Check sheet for the modelled part. Datum: model origin and axes. Units: mm. A direction names the side the tool comes from. Round coordinates to 2 decimals unless told otherwise and drop trailing zeros. Loops run counter-clockwise (first coordinate to the right, second up) from the corner with the lowest first, then second, coordinate; pieces in that order, holes last. Notation, with made-up numbers: (80, 67) - (111, 67) arc R14 ccw to (111, 90) - close; hole circle Ø3 at (61.5, 43). An arc over 180 degrees is marked (long way). Answer in a Markdown table with one row per item. Add a question column.
(1) Access from +Z, -Z, +X, -X, +Y, -Y to the whole of each face (thin tool, end or side, straight path). Record for faces 1 (the cylindrical face through (1, 1.05, 4.03)), 2 (the flat face through (19.8, 35, 3.5)).
(2) Thickness scan on line 1 along Y through (x, z) = (36.5, 3.65); line 2 along Y through (x, z) = (18, 5.55); line 3 along X through (y, z) = (32, 3.55). Record the ranges inside material, lowest first.
(3) Gauge pin test, flat end, axial feed: pin 1 (0.9 mm diameter, centred on x = 37, y = 36, fed in from +Z). Record the tip position at first contact, or that the pin passes through.
(4) Cross-section at B-B on x = 21.5. Enter the section's corners in (y, z).
(5) Cross-section at A-A on z = 4.5. Count the separate pieces of the cut face and the enclosed holes in it, then the cut area to 3 significant figures.
(6) Mould release check, pull along X, two halves, no side actions. Record for faces 3 (the flat face through (36, 37, 2)), 4 (the flat face through (20, 0, 4)), 5 (the cylindrical face through (1, 38.95, 3.97)): +X half, -X half, draft (parallel to the pull), parting line (faces both ways), or undercut.
(7) Cross-section at C-C on y = 6. Enter the section's corners in (x, z).
from build123d import *

# Parameters (mm, degrees)
SKETCH1_W           = 40
SKETCH1_H           = 40
BOSS_EXTRUDE1_DEPTH = 2
SKETCH2_W           = 40
SKETCH2_H           = 40
SKETCH2_W_2         = 30
SKETCH2_H_2         = 30
BOSS_EXTRUDE2_DEPTH = 2
SKETCH3_W           = 40
SKETCH3_H           = 40
SKETCH3_W_2         = 32
SKETCH3_H_2         = 32
BOSS_EXTRUDE3_DEPTH = 2
SKETCH4_R           = 1.5
CUT_EXTRUDE1_DEPTH  = 4
FILLET1_R           = 3.5
FILLET2_R           = 2


with BuildPart() as part:
    # Sketch1 → Boss-Extrude1 (new body)
    with BuildSketch(Plane.XY):
        with Locations((20, 20)):
            Rectangle(SKETCH1_W, SKETCH1_H)
    extrude(amount=BOSS_EXTRUDE1_DEPTH)

    # Sketch2 → Boss-Extrude2 (add)
    with BuildSketch(Plane.XY.offset(2)):
        with Locations((20, 20)):
            Rectangle(SKETCH2_W, SKETCH2_H)
        with Locations((20, 20)):
            Rectangle(SKETCH2_W_2, SKETCH2_H_2, mode=Mode.SUBTRACT)
    extrude(amount=BOSS_EXTRUDE2_DEPTH)

    # Sketch3 → Boss-Extrude3 (add)
    # profile 1 of 5: a face of its own
    with BuildSketch(Plane.XY.offset(4)):
        with Locations((20, 20)):
            Rectangle(SKETCH3_W, SKETCH3_H)
        with Locations((20, 20)):
            Rectangle(SKETCH3_W_2, SKETCH3_H_2, mode=Mode.SUBTRACT)
    # profile 2 of 5: a face of its own
    with BuildSketch(Plane.XY.offset(4)):
        Polygon((15, 36), (4, 36), (4, 25), (5, 25), (5, 35), (15, 35), align=None)
    # profile 3 of 5: a face of its own
    with BuildSketch(Plane.XY.offset(4)):
        Polygon((36, 36), (25, 36), (25, 35), (35, 35), (35, 25), (36, 25), align=None)
    # profile 4 of 5: a face of its own
    with BuildSketch(Plane.XY.offset(4)):
        Polygon((36, 4), (36, 15), (35, 15), (35, 5), (25, 5), (25, 4), align=None)
    # profile 5 of 5: a face of its own
    with BuildSketch(Plane.XY.offset(4)):
        Polygon((5, 15), (4, 15), (4, 4), (15, 4), (15, 5), (5, 5), align=None)
    extrude(amount=BOSS_EXTRUDE3_DEPTH)

    # Sketch4 → Cut-Extrude1 (cut)
    with BuildSketch(Plane.XY.offset(6)):
        with Locations((3.5, 36.5)):
            Circle(SKETCH4_R)
        with Locations((36.5, 36.5)):
            Circle(SKETCH4_R)
        with Locations((36.5, 3.5)):
            Circle(SKETCH4_R)
        with Locations((3.5, 3.5)):
            Circle(SKETCH4_R)
    extrude(amount=-CUT_EXTRUDE1_DEPTH, mode=Mode.SUBTRACT)

    # Fillet1
    fillet1_edges = [part.edges().sort_by_distance(p)[0] for p in [
        (0, 40, 3),
        (40, 40, 3),
        (40, 0, 3),
        (0, 0, 3),
    ]]
    fillet(fillet1_edges, radius=FILLET1_R)

    # Fillet2
    fillet2_edges = [part.edges().sort_by_distance(p)[0] for p in [
        (20, 0, 0),
        (0, 20, 0),
        (20, 40, 0),
        (40, 20, 0),
        (1.025126266, 38.974873734, 0),
        (38.974873734, 38.974873734, 0),
        (38.974873734, 1.025126266, 0),
        (1.025126266, 1.025126266, 0),
    ]]
    fillet(fillet2_edges, radius=FILLET2_R)


solid = part.part
Answers:
| question | item | result |
|---|---|---|
| 1 | face 1 | +Z, -Z, -X, -Y |
| 1 | face 2 | +Z |
| 2 | line 1 | y = 0 to 2, 5 to 35, 38 to 40 |
| 2 | line 2 | y = 0 to 4, 36 to 40 |
| 2 | line 3 | x = 0 to 5, 35 to 40 |
| 3 | pin 1 | stops at z = 2 |
| 4 | outline | (0, 2) arc R2 ccw to (2, 0) - (38, 0) arc R2 ccw to (40, 2) - (40, 6) - (36, 6) - (36, 4) - (35, 4) - (35, 2) - (5, 2) - (5, 4) - (4, 4) - (4, 6) - (0, 6) - close |
| 5 | separate pieces | 1 |
| 5 | enclosed holes | 5 |
| 5 | area | 621 mm^2 |
| 6 | face 3 | undercut |
| 6 | face 4 | draft |
| 6 | face 5 | -X half |
| 7 | outline | (0, 2) arc R2 ccw to (2, 0) - (38, 0) arc R2 ccw to (40, 2) - (40, 6) - (35, 6) - (35, 2) - (5, 2) - (5, 6) - (0, 6) - close |
